Check sheet for the drawn part. Datum: minimum x, y, z corner. Units: mm. A direction names the side the tool comes from. Coordinates: 2 decimals unless noted, no trailing zeros. Order: outer loops, then holes, each group sorted by start corner. A loop starts at its lowest first (then second) coordinate and runs counter-clockwise, first axis right, second up.
Q1. Thickness scan on line 1 (Y direction, x = 5.65, z = 49.75); line 2 (Z direction, x = 33.3, y = 47.6); line 3 (Y direction, x = 28, z = 42). Record the ranges inside material, lowest first.
Q2. Cross-section at D-D, the plane x = 24. Record the boundary of the cut face in (y, z), and give its area (3 significant figures).
Q3. Cross-section at A-A, the plane y = 5.65. Record the boundary of the cut face in (x, z).
Q4. Cross-section at B-B, the plane x = 36.65. Record the boundary of the cut face in (y, z).
Q5. Depth check by flat-ended pin: P1, Ø9, axis at y = 42.5, z = 18.5, coming from the -X side; P2, Ø3.5, axis at x = 19, y = 46.5, coming from the -Z side; P3, Ø12, axis at x = 35, y = 27, coming from the -Z side. Enter the tip coordinate at first touch or a pass-through.
Q6. Cross-section at C-C, the plane z = 4.5. Record the boundary of the cut face in (x, y), and give its area (3 significant figures).
Q7. Set-up check for the marked faces 1 and 2: record each of +Z, -Z, +X, -X, +Y, -Y from which the full face is reachable in a straight line by a thin tool's end or side.
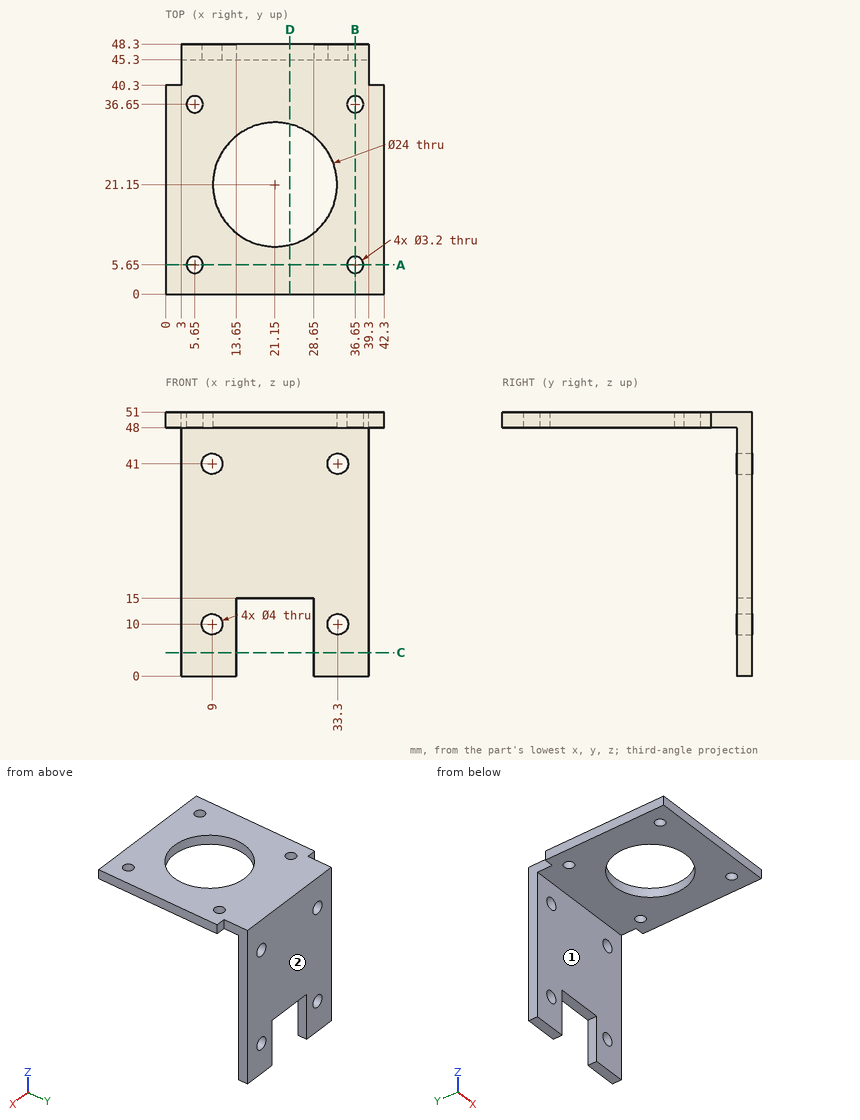
Check values:
1. line 1: y = 0 to 4.05, 7.25 to 35.05, 38.25 to 48.3
1. line 2: z = 0 to 8, 12 to 39, 43 to 51
1. line 3: y = 45.3 to 48.3
2. outline: (0, 48) - (9.49, 48) - (9.49, 51) - (0, 51) - close; (32.81, 48) - (45.3, 48) - (45.3, 15) - (48.3, 15) - (48.3, 51) - (32.81, 51) - close
2. area: 174 mm2
3. outline: (0, 48) - (4.05, 48) - (4.05, 51) - (0, 51) - close; (7.25, 48) - (35.05, 48) - (35.05, 51) - (7.25, 51) - close; (38.25, 48) - (42.3, 48) - (42.3, 51) - (38.25, 51) - close
4. outline: (0, 48) - (4.05, 48) - (4.05, 51) - (0, 51) - close; (7.25, 48) - (35.05, 48) - (35.05, 51) - (7.25, 51) - close; (38.25, 48) - (45.3, 48) - (45.3, 0) - (48.3, 0) - (48.3, 51) - (38.25, 51) - close
5. P1: stops at x = 3
5. P2: stops at z = 15
5. P3: stops at z = 48
6. outline: (3, 45.3) - (13.65, 45.3) - (13.65, 48.3) - (3, 48.3) - close; (28.65, 45.3) - (39.3, 45.3) - (39.3, 48.3) - (28.65, 48.3) - close
6. area: 63.9 mm2
7. face 1: -Z, +X, -X, -Y
7. face 2: +Z, -Z, +X, -X, +Y
